Autodesk Inventor part; units mm, degrees
ref_plane "YZ Plane" through (0, 0, 0) normal (1, 0, 0) x (0, 1, 0)
ref_plane "XZ Plane" through (0, 0, 0) normal (0, 1, 0) x (-1, 0, 0)
ref_plane "XY Plane" through (0, 0, 0) normal (0, 0, 1) x (1, 0, 0)
sketch "Sketch1" plane through (0, 0, 0) normal (0, 1, 0) x (-1, 0, 0)
  line L0 (0, 0) -> (139.342, 0)
  line L1 (139.342, 0) -> (139.342, -147.342)
  line L2 (139.342, -147.342) -> (0, -147.342)
  line L3 (0, -147.342) -> (0, 0)
  line L4 (139.342, -147.342) -> (142.342, -147.342)
  line L5 (142.342, -147.342) -> (142.342, 0)
  line L6 (142.342, 0) -> (139.342, 0)
  line L7 (0, 0) -> (-3, 0)
  line L8 (-3, 0) -> (-3, -147.342)
  line L9 (-3, -147.342) -> (0, -147.342)
  dimension "d0" = 139.342
  dimension "d1" = 147.342
  dimension "d2" = 3
  dimension "d3" = 3
extrude "Extrusion1" add sketch "Sketch1" along normal blind 15 contours L3 L9 L8 L7 | L6 L5 L4 L1
sketch "Sketch2" plane through (-139.342, 0, 0) normal (1, 0, 0) x (0, 0, -1)
  point P0 (0, 0)
sketch "Sketch3" plane through (0, 15, 0) normal (0, 1, 0) x (1, 0, 0)
  point P0 (0, 0)
sketch "Sketch4" plane through (0, 15, 0) normal (0, 1, 0) x (1, 0, 0)
  line L0 (-139.342, 147.342) -> (-142.342, 147.342)
  line L1 (0, 0) -> (3, 0)
  line L2 (-142.342, 147.342) -> (3, 147.342)
  line L3 (3, 147.342) -> (3, 0)
  line L4 (3, 0) -> (-142.342, 0)
  line L5 (-142.342, 0) -> (-142.342, 147.342)
extrude "Extrusion2" add sketch "Sketch4" along normal blind 12.5
chamfer "Chamfer1" distance 14.75 angle 45 1 edges at (-69.671, 27.5, -147.342)
sketch "Sketch5" plane through (3, 0, 0) normal (1, 0, 0) x (0, 0, -1)
  line L0 (132.592, 27.5) -> (147.342, 12.75)
  arc A0 (132.592, 27.5) -> (0, 27.5) centre (66.296, -181.534) ccw
  line L1 (0, 27.5) -> (132.592, 27.5)
  point P0 (0, 0)
extrude "Extrusion3" add sketch "Sketch5" against normal blind 145.342
sketch "Sketch6" plane through (-142.342, 0, -147.342) normal (-1, 0, 0) x (0, 0, 1)
  line L0 (147.342, 0) -> (147.342, 27.5)
  line L1 (147.342, 0) -> (147.342, 15)
  line L2 (0, 12.75) -> (14.75, 27.5)
  line L3 (147.342, 15) -> (0, 12.75)
  line L4 (0, 12.75) -> (1.9998, 12.7805)
  line L5 (1.9998, 12.7805) -> (15.7346, 26.5154)
  line L6 (147.342, 15) -> (145.3422, 14.9695)
  line L7 (145.3422, 14.9695) -> (145.1659, 26.5154)
  arc A0 (145.1659, 26.5154) -> (15.7346, 26.5154) centre (80.4503, -220.3584) ccw
  dimension "d13" = 15
  dimension "d14" = 2
  dimension "d15" = 2
extrude "Extrusion4" cut sketch "Sketch6" against normal blind 142.342
sketch "Sketch7" plane through (-142.342, 0, -147.342) normal (-1, 0, 0) x (0, 0, 1)
  line L0 (1.9998, 12.7805) -> (145.3422, 14.9695)
  arc A0 (145.1659, 26.5154) -> (15.7346, 26.5154) centre (80.4503, -220.3584) ccw
  line L1 (1.9998, 12.7805) -> (15.7346, 26.5154)
  line L2 (145.1659, 26.5154) -> (145.3418, 15)
  line L3 (145.1659, 26.5154) -> (145.3418, 15)
  line L4 (145.3418, 15) -> (145.3418, 15)
  line L5 (1.9998, 12.7805) -> (145.3418, 15)
  arc A1 (145.1659, 26.5154) -> (15.7346, 26.5154) centre (80.4503, -220.3584) ccw
  point P0 (147.342, 0)
extrude "Extrusion5" add sketch "Sketch7" against normal blind 3.002
properties part number "El capo"
The listing builds one solid part. Answer for the finished solid, in the listing's coordinates (mm). A direction names the side the tool comes from. Round coordinates to 2 decimals unless told otherwise and drop trailing zeros. Order: outer loops, then holes, each group sorted by start corner. A loop starts at its lowest first (then second) coordinate and runs counter-clockwise, first axis right, second up. Notation, with made-up numbers: M 66.25,89.25 L 109.25,89.25 A19 cw 109.25,96.25 Z; hole C 43.5,-15 d2. An arc over 180 degrees is marked long. Answer in a Markdown table with one row per item. Add a question column.
1) Consider line 1 along X through (y, z) = (6, -83); line 2 along Z through (x, y) = (-14, 18.5); line 3 along Z through (x, y) = (-27.5, 19). Determine where each line is inside the solid, lowest interval first. Write a range as from..to.
2) Flat-ended cylindrical pins translate along their axes: pin 1 Ø2 at (x, z) = (-13, -38.5) entering from +Y; pin 2 Ø2 at (x, z) = (-37.5, -27.5) entering from +Y; pin 3 Ø0.6 at (x, z) = (-49, -144.5) entering from -Y. Find the tip coordinate at first contact, or state that the pin passes through.
3) The part is cut by section C-C on z = -42. Determine the outline of the cut face in (x, y), plus the area to 3 significant figures.
4) The part is cut by section A-A on y = 10.5. Determine the outline of the cut face in (x, z), plus the area to 3 significant figures.
5) The part is cut by section B-B on x = -39.5. Determine the outline of the cut face in (y, z).
6) Which of the six approach directions +Z, -Z, +X, -X, +Y, -Y give full straight-line access (tool end or side, diameter ignored) to faces 1 (the face through (3, 19, -75)), 2 (the face through (0, 17, -75)), 3 (the face through (-139.342, 7, -73))?
7) The part is cut by section D-D on y = 18.5. Determine the outline of the cut face in (x, z), plus the area to 3 significant figures.
8) Determine the mould class of faces 4 (the face through (-70.645, 34.855, -65.976)), 5 (the face through (-70.69, 21.66, -138.43)), 6 (the face through (-142.342, 19, -73)) for opening direction Z: pulls with the +Z half, pulls with the -Z half, needs draft (parallel to the pull), parting line crosses it, or undercut.
Findings below:
| question | item | result |
|---|---|---|
| 1 | line 1 | x = -142.34..-139.34, 0..3 |
| 1 | line 2 | z = -141.59..-139.62, -2.05..0 |
| 1 | line 3 | z = -141.09..-139.12, -2.06..0 |
| 2 | pin 1 | stops at y = 36.12 |
| 2 | pin 2 | stops at y = 34.48 |
| 2 | pin 3 | stops at y = 15 |
| 3 | outline | M -142.34,0 L -139.34,0 L -139.34,14.36 L -142.34,14.36 Z; M -142.34,14.38 L -139.34,14.38 L -139.34,33.64 L 0,33.64 L 0,0 L 3,0 L 3,36.41 L -142.34,36.41 Z |
| 3 | area | 605 mm² |
| 4 | outline | M -142.34,-147.34 L -139.34,-147.34 L -139.34,0 L -142.34,0 Z; M 0,-147.34 L 3,-147.34 L 3,0 L 0,0 Z |
| 4 | area | 884 mm² |
| 5 | outline | M 15,-145.09 L 27.5,-132.59 A219.3 ccw 27.5,0 L 15,0 L 15,-2 L 26.52,-2.18 A255.22 cw 26.52,-131.61 L 15,-143.12 Z |
| 6 | face 1 | +Z, -Z, +X, +Y, -Y |
| 6 | face 2 | -Y |
| 6 | face 3 | +Z, -Z, -Y |
| 7 | outline | M -142.34,-141.59 L 3,-141.59 L 3,0 L -142.34,0 Z; hole M -139.34,-139.62 L 0,-139.62 L 0,-2.05 L -139.34,-2.05 Z |
| 7 | area | 1,410 mm² |
| 8 | face 4 | undercut |
| 8 | face 5 | pulls with the -Z half |
| 8 | face 6 | needs draft |
